Geometry check sheet. Reference: the model listing, model coordinates, mm. A direction names the side the tool comes from. Coordinates: 2 decimals unless noted, no trailing zeros. Write each loop counter-clockwise with the first axis right and the second up, starting at its lowest first coordinate (ties: lowest second). Pieces come first, ordered by that corner, then holes. Notation, with made-up numbers: (67.5, 10) -> (82.5, 10) arc R18 cw to (82.5, 27) -> close; hole circle Ø8 at (-18, 31). An arc over 180 degrees is marked (long way). Use a Markdown table: item, result.
```python
from build123d import *

# Parameters (mm, degrees)
F1_DEPTH = 90
F3_D     = 4.4
F3_DEPTH = 12
F3_TIP   = 1.3218933619
F4_R     = 5
F6_DEPTH = 0.46
F7_R     = 1
F9_D     = 4.4
F9_DEPTH = 12
F9_TIP   = 1.3218933619


with BuildPart() as f1:
    # F0 (on Front) → F1 (new body)
    with BuildSketch(Plane.XZ):
        with BuildLine():
            Line((-25, -25), (25, -25))
            Line((25, -25), (25, 0))
            Line((25, 0), (16, 0))
            ThreePointArc((16, 0), (0, -16), (-16, 0))
            Line((-16, 0), (-25, 0))
            Line((-25, 0), (-25, -25))
        make_face()
    extrude(amount=F1_DEPTH)

    # F3
    with Locations(Plane.XY):
        with Locations((-20, -5), (20, -5), (20, -85), (-20, -85)):
            Hole(F3_D / 2, depth=F3_DEPTH)
            with Locations((0, 0, -(F3_DEPTH + F3_TIP / 2))):  # 118° drill point
                Cone(0, F3_D / 2, F3_TIP, mode=Mode.SUBTRACT)

    # F4
    f4_edges = [f1.edges().sort_by_distance(p)[0] for p in [
        (0, -90, -16),
    ]]
    fillet(f4_edges, radius=F4_R)

    # F5 (on face) → F6 (cut)
    with BuildSketch(Plane.XY):
        Polygon((-16, -42.614615115), (-16, -64.914615115), (31.2709680734, -39.7801955466), (31.2709680734, -17.4801955466), align=None)
        Polygon((-25, -47.4), (-25, -69.7), (-16, -64.914615115), (-16, -42.614615115), align=None)
    extrude(amount=-F6_DEPTH, mode=Mode.SUBTRACT)

    # F7
    f7_edges = [f1.edges().sort_by_distance(p)[0] for p in [
        (25, -90, -12.5),
        (25, -45, -25),
        (25, 0, -12.5),
        (0, -90, -25),
        (-25, -90, -12.5),
        (0, 0, -25),
        (-25, 0, -12.5),
        (-25, -45, -25),
    ]]
    fillet(f7_edges, radius=F7_R)

    # F9
    with Locations(Plane(origin=(0, 0, -25), x_dir=(1, 0, 0), z_dir=(0, 0, -1))):
        with Locations((20, 30), (-20, 30), (-20, 60), (20, 60)):
            Hole(F9_D / 2, depth=F9_DEPTH)
            with Locations((0, 0, -(F9_DEPTH + F9_TIP / 2))):  # 118° drill point
                Cone(0, F9_D / 2, F9_TIP, mode=Mode.SUBTRACT)


solid = f1.part
```
Item 1: Thickness scan on L1, parallel to Y at x = 20, z = -8.75; L2, parallel to X at y = -30, z = -18.75; L3, parallel to Y at x = 20, z = -19.75. Record the ranges inside material, lowest first. Write a range as [from, to].
Answer block:
| item | result |
|---|---|
| L1 | y = [-90, -87.2], [-82.8, -7.2], [-2.8, 0] |
| L2 | x = [-25, -22.2], [-17.8, 17.8], [22.2, 25] |
| L3 | y = [-90, -62.2], [-57.8, -32.2], [-27.8, 0] |
Item 2: Section check A-A on y = -63.5. Record the boundary of the cut face in (x, z).
Answer block:
| item | result |
|---|---|
| outline | (-25, -24) arc R1 ccw to (-24, -25) -> (24, -25) arc R1 ccw to (25, -24) -> (25, 0) -> (16, 0) arc R16 cw to (-15.99, -0.46) -> (-25, -0.46) -> close |
Item 3: Section check C-C on y = -11. Record the boundary of the cut face in (x, z).
Answer block:
| item | result |
|---|---|
| outline | (-25, -24) arc R1 ccw to (-24, -25) -> (24, -25) arc R1 ccw to (25, -24) -> (25, 0) -> (16, 0) arc R16 cw to (-16, 0) -> (-25, 0) -> close |
Item 4: Tool access check on faces 1 (the cylindrical face through (-21.02, -28.05, -18.92)), 2 (the flat face through (0, 0, -17)), 3 (the flat face through (-21, -56, -0.46)). Record the directions out of +Z, -Z, +X, -X, +Y, -Y that give a thin tool (end or side, any length) a straight path to the whole face; none if there is none.
Answer block:
| item | result |
|---|---|
| face 1 | -Z |
| face 2 | +Z, -Z, +X, -X, +Y |
| face 3 | +Z |
Item 5: Mould release check, pull along Y, two halves, no side actions. Record for faces 4 (the flat face through (0, -90, -22)), 5 (the cylindrical face through (18.98, -58.05, -18.92)), 6 (the flat face through (-25, -44, -12)): +Y half, -Y half, draft (parallel to the pull), parting line (faces both ways), or undercut.
Answer block:
| item | result |
|---|---|
| face 4 | -Y half |
| face 5 | undercut |
| face 6 | draft |
Item 6: Depth check by flat-ended pin: P1, Ø2.5, axis at x = 22.5, y = -40, coming from the +Z side; P2, Ø3, axis at x = 9.5, z = -12, coming from the -Y side; P3, Ø1.5, axis at x = -1.5, y = -51.5, coming from the +Z side. Enter the tip coordinate at first touch or a pass-through.
Answer block:
| item | result |
|---|---|
| P1 | stops at z = -0.46 |
| P2 | stops at y = -87.72 |
| P3 | stops at z = -15.84 |
Item 7: Section check B-B on z = -5. Count the separate pieces of the cut face and the enclosed holes in it, then the cut area to 3 significant figures.
Answer block:
| item | result |
|---|---|
| separate pieces | 2 |
| enclosed holes | 4 |
| area | 1,690 mm^2 |
